```python
from build123d import *

# Parameters (mm, degrees)
SKETCH1_R                  = 57
EXTRUDE4_DEPTH             = 7.5
SKETCH_R                   = 60
SKETCH_R_2                 = 57
EXTRUDE5_DEPTH             = 5
EXTRUDE6_DEPTH             = 86.183625187
EXTRUDE6_DEPTH_BACK        = 86.183625187
SKETCH5_R                  = 18
F_4_5_4_5_DIAMETER_HOLE1_D = 4.5
CIRPATTERN1_COUNT          = 4
M5_CLEARANCE_HOLE1_D       = 5.5


with BuildPart() as part:
    # Sketch1 → Extrude4 (new, symmetric)
    with BuildSketch(Plane(origin=(0, 0, 0), x_dir=(1, 0, 0), z_dir=(0, 1, 0))):
        with Locations(Location((0, 0, 0), (0, 0, 270))):
            Circle(SKETCH1_R)
    extrude(amount=EXTRUDE4_DEPTH, both=True)

    # Sketch → Extrude5 (add, symmetric)
    with BuildSketch(Plane(origin=(0, 0, 0), x_dir=(1, 0, 0), z_dir=(0, 1, 0))):
        with Locations(Location((0, 0, 0), (0, 0, 270))):
            Circle(SKETCH_R)
        with Locations(Location((0, 0, 0), (0, 0, 270))):
            Circle(SKETCH_R_2, mode=Mode.SUBTRACT)
    extrude(amount=EXTRUDE5_DEPTH, both=True)

    # Sketch5 → Extrude6 (cut, two sides: drawn at the far end of the back side and taken through both)
    with BuildSketch(Plane(origin=(0, 0, 0), x_dir=(1, 0, 0), z_dir=(0, 1, 0)).offset(-EXTRUDE6_DEPTH_BACK)):
        with Locations(Location((0, 0, 0), (0, 0, 270))):
            Circle(SKETCH5_R)
    extrude(amount=EXTRUDE6_DEPTH + EXTRUDE6_DEPTH_BACK, mode=Mode.SUBTRACT)

    # 4.5 _4.5_ Diameter Hole1 (through all)
    with Locations(Plane(origin=(0, -7.5, 0), x_dir=(-1, 0, 0), z_dir=(0, -1, 0))):
        with Locations((15.556349186, 15.556349186)):
            f_4_5_4_5_diameter_hole1 = Hole(F_4_5_4_5_DIAMETER_HOLE1_D / 2)

    # CirPattern1: 4.5 _4.5_ Diameter Hole1 ×4 about axis
    cirpattern1_axis = Axis((0, 0, 0), (0, 1, 0))
    for i in range(1, CIRPATTERN1_COUNT):
        add(f_4_5_4_5_diameter_hole1.rotate(cirpattern1_axis, i * 360 / CIRPATTERN1_COUNT), mode=Mode.SUBTRACT)

    # M5 Clearance Hole1 (through all)
    with Locations(Plane(origin=(0, 7.5, 0), x_dir=(1, 0, 0), z_dir=(0, 1, 0))):
        with Locations((-37.5, 18), (-37.5, -18)):
            Hole(M5_CLEARANCE_HOLE1_D / 2)


solid = part.part
```
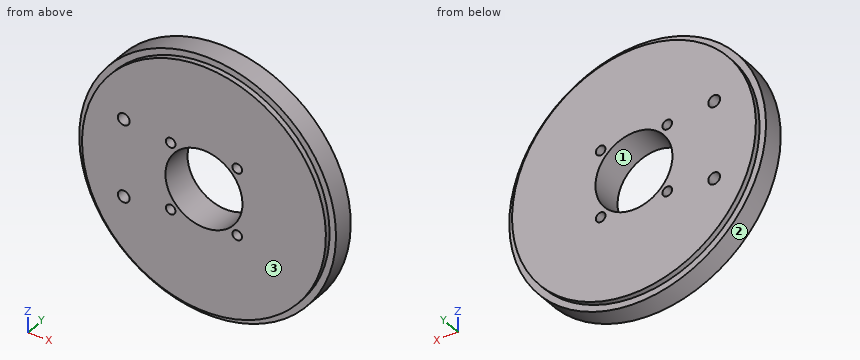
Could you check a few things on this model? Use its own coordinates, in mm. Face numbers are marked on the shaded views. Round coordinates to 2 decimals unless told otherwise and drop trailing zeros. Loops run counter-clockwise (first coordinate to the right, second up) from the corner with the lowest first, then second, coordinate; pieces in that order, holes last. Notation, with made-up numbers: (13, -17.75) - (22, -17.75) arc R31 cw to (22, 9.25) - close; hole circle Ø5 at (37, -11.75). An arc over 180 degrees is marked (long way). Answer as CSV lines item,"result".
1. Please list where these lines run through material, in increasing order: line 1 along Z through (x, y) = (-37.5, 1); line 2 along X through (y, z) = (-2.5, -1); line 3 along X through (y, z) = (3.25, -19). Write a range as [from, to].
Filled in:
line 1,"z = [-46.84, -20.75], [-15.25, 15.25], [20.75, 46.84]"
line 2,"x = [-59.99, -17.97], [17.97, 59.99]"
line 3,"x = [-56.91, -40.06], [-34.94, 56.91]"
2. For pin 1 Ø3 at (y, z) = (4.5, 39.5) entering from -X; pin 2 Ø1.5 at (y, z) = (2.5, -17.5) entering from -X; pin 3 Ø6 at (y, z) = (-5.5, 45.5) entering from +X, each with a flat end and sliding along its axis, tell me the tip position at first contact or that it passes through.
Filled in:
pin 1,"stops at x = -46.43"
pin 2,"stops at x = -57.61"
pin 3,"stops at x = 42.31"
3. I want a section at A-A on x = 0. List the corners of the cut face in (y, z) for me.
Filled in:
outline,"(-7.5, -57) - (-5, -57) - (-5, -60) - (5, -60) - (5, -57) - (7.5, -57) - (7.5, -18) - (-7.5, -18) - close; (-7.5, 18) - (7.5, 18) - (7.5, 57) - (5, 57) - (5, 60) - (-5, 60) - (-5, 57) - (-7.5, 57) - close"
4. I want a section at B-B on z = 0. List the corners of the cut face in (x, y) for me, then the cut area to 3 significant figures.
Filled in:
outline,"(-60, -5) - (-57, -5) - (-57, -7.5) - (-18, -7.5) - (-18, 7.5) - (-57, 7.5) - (-57, 5) - (-60, 5) - close; (18, -7.5) - (57, -7.5) - (57, -5) - (60, -5) - (60, 5) - (57, 5) - (57, 7.5) - (18, 7.5) - close"
area,"1,230 mm^2"
5. We'd pull the mould along X, two halves only. Please class the marked faces 1, 2 and 3: +X half, -X half, draft (parallel to the pull), parting line (faces both ways), or undercut.
Filled in:
face 1,"undercut"
face 2,"parting line"
face 3,"draft"
6. I want a section at D-D on x = -37.5. List the corners of the cut face in (y, z) for me.
Filled in:
outline,"(-7.5, -42.93) - (-5, -42.93) - (-5, -46.84) - (5, -46.84) - (5, -42.93) - (7.5, -42.93) - (7.5, -20.75) - (-7.5, -20.75) - close; (-7.5, -15.25) - (7.5, -15.25) - (7.5, 15.25) - (-7.5, 15.25) - close; (-7.5, 20.75) - (7.5, 20.75) - (7.5, 42.93) - (5, 42.93) - (5, 46.84) - (-5, 46.84) - (-5, 42.93) - (-7.5, 42.93) - close"
7. I want a section at C-C on y = -0.5. List the corners of the cut face in (x, z) for me, then the cut area to 3 significant figures.
Filled in:
outline,"circle Ø120 at (0, 0); hole circle Ø5.5 at (-37.5, -18); hole circle Ø5.5 at (-37.5, 18); hole circle Ø36 at (0, 0); hole circle Ø4.5 at (-15.56, -15.56); hole circle Ø4.5 at (-15.56, 15.56); hole circle Ø4.5 at (15.56, -15.56); hole circle Ø4.5 at (15.56, 15.56)"
area,"10,200 mm^2"
